Source: CAD feature listing. Evaluate the final solid. Frame: model axes, mm. Coordinates: 2 decimals unless noted, no trailing zeros. Loops run counter-clockwise (first coordinate to the right, second up) from the corner with the lowest first, then second, coordinate; pieces in that order, holes last.
```python
from build123d import *

# Parameters (mm, degrees)
SKETCH2_R           = 5
BOSS_EXTRUDE1_DEPTH = 10
FILLET1_R           = 3
BOSS_EXTRUDE2_DEPTH = 10
SKETCH4_R           = 1.5
CUT_EXTRUDE1_DEPTH  = 14


with BuildPart() as part:
    # Sketch2 → Boss-Extrude1 (new body)
    with BuildSketch(Plane(origin=(0, 0, 0), x_dir=(1, 0, 0), z_dir=(0, 1, 0))):
        with BuildLine():
            Line((36.25, 10), (-36.25, 10))
            ThreePointArc((-36.25, 10), (-46.25, 0), (-36.25, -10))
            Line((-36.25, -10), (36.25, -10))
            ThreePointArc((36.25, -10), (46.25, 0), (36.25, 10))
        make_face()
        with Locations((-36.25, 0)):
            Circle(SKETCH2_R, mode=Mode.SUBTRACT)
        with BuildLine():
            ThreePointArc((5, 0), (3.535533906, -3.535533906), (0, -5))
            ThreePointArc((0, -5), (-5, 0), (0, 5))
            ThreePointArc((0, 5), (3.535533906, 3.535533906), (5, 0))
        make_face(mode=Mode.SUBTRACT)
        with Locations((36.25, 0)):
            Circle(SKETCH2_R, mode=Mode.SUBTRACT)
    extrude(amount=BOSS_EXTRUDE1_DEPTH)

    # Fillet1
    fillet1_edges = [part.edges().sort_by_distance(p)[0] for p in [
        (46.25, 0, 0),
        (0, 0, 10),
        (0, 10, 10),
        (46.25, 10, 0),
        (0, 10, -10),
        (-46.25, 10, 0),
        (-46.25, 0, 0),
        (0, 0, -10),
    ]]
    fillet(fillet1_edges, radius=FILLET1_R)

    # Sketch3 → Boss-Extrude2 (add)
    with BuildSketch(Plane(origin=(0, 10, 0), x_dir=(1, 0, 0), z_dir=(0, 1, 0))):
        with BuildLine():
            Line((5, 0), (0, 0))
            Line((0, 0), (-5, 0))
            ThreePointArc((-5, 0), (0, -5), (5, 0))
        make_face()
        with BuildLine():
            Line((-5, 0), (0, 0))
            Line((0, 0), (5, 0))
            ThreePointArc((5, 0), (0, 5), (-5, 0))
        make_face()
    extrude(amount=-BOSS_EXTRUDE2_DEPTH)

    # Sketch4 → Cut-Extrude1 (cut)
    with BuildSketch(Plane(origin=(0, 10, 0), x_dir=(1, 0, 0), z_dir=(0, 1, 0))):
        with Locations((-6.5, 0)):
            Circle(SKETCH4_R)
        with Locations((6.5, 0)):
            Circle(SKETCH4_R)
    extrude(amount=-CUT_EXTRUDE1_DEPTH, mode=Mode.SUBTRACT)


solid = part.part
```
Q1. Section query C-C on y = 8.5. Return the cut outline in (x, z), then the cut area to 3 significant figures.
Q2. Draft query along X for faces 1 (the cylindrical face through (-8, 5, 0)), 2 (the cylindrical face through (0.51, 0.9, 9.14)), 3 (the cylindrical face through (46.248, 4.972, 0.22)), 4 (the cylindrical face through (-46.248, 4.972, -0.22)). Return one class per face: released by +X, released by -X, zero draft, split by the parting line, or undercut.
Q3. Section query B-B on x = 6.5. Return the cut outline in (y, z).
Q4. Material intervals for line 1 along X through (y, z) = (4, 0); line 2 along X through (y, z) = (0.5, -3.75); line 3 along Z through (x, y) = (6.5, 4), sorted ascending.
Q5. First-contact query: pin 1 Ø1 at (y, z) = (3, 3.5) entering from -X; pin 2 Ø3 at (y, z) = (2, -3) entering from +X; pin 3 Ø1.5 at (y, z) = (4, 3) entering from -X. Flat tips, straight axial feed; report the tip coordinate or a pass-through.
Q6. Section query A-A on z = 0. Return the cut outline in (x, y), then the cut area to 3 significant figures.
Resolved:
1. outline: (-36.25, -9.6) - (36.25, -9.6) arc R9.6 ccw to (36.25, 9.6) - (-36.25, 9.6) arc R9.6 ccw to start; hole circle Ø10 at (-36.25, 0); hole circle Ø3 at (-6.5, 0); hole circle Ø3 at (6.5, 0); hole circle Ø10 at (36.25, 0)
1. area: 1,510 mm2
2. face 1: undercut
2. face 2: zero draft
2. face 3: released by +X
2. face 4: released by -X
3. outline: (0, -7) arc R3 ccw to (3, -10) - (7, -10) arc R3 ccw to (10, -7) - (10, -1.5) - (0, -1.5) - close; (0, 1.5) - (10, 1.5) - (10, 7) arc R3 ccw to (7, 10) - (3, 10) arc R3 ccw to (0, 7) - close
4. line 1: x = -46.25 to -41.25, -31.25 to -8, -5 to 5, 8 to 31.25, 41.25 to 46.25
4. line 2: x = -44.05 to -39.56, -32.94 to 32.94, 39.56 to 44.05
4. line 3: z = -10 to -1.5, 1.5 to 10
5. pin 1: stops at x = -45.79
5. pin 2: stops at x = 46.09
5. pin 3: stops at x = -45.99
6. outline: (-46.25, 3) arc R3 ccw to (-43.25, 0) - (-41.25, 0) - (-41.25, 10) - (-43.25, 10) arc R3 ccw to (-46.25, 7) - close; (-31.25, 0) - (-8, 0) - (-8, 10) - (-31.25, 10) - close; (-5, 0) - (5, 0) - (5, 10) - (-5, 10) - close; (8, 0) - (31.25, 0) - (31.25, 10) - (8, 10) - close; (41.25, 0) - (43.25, 0) arc R3 ccw to (46.25, 3) - (46.25, 7) arc R3 ccw to (43.25, 10) - (41.25, 10) - close
6. area: 657 mm2
